The listing builds one solid part. Answer for the finished solid, in the listing's coordinates (mm). A direction names the side the tool comes from. Coordinates: 2 decimals unless noted, no trailing zeros. Order: outer loops, then holes, each group sorted by start corner. A loop starts at its lowest first (then second) coordinate and runs counter-clockwise, first axis right, second up. Notation, with made-up numbers: (-0.5, -6) -> (39.5, -6) arc R35 cw to (39.5, 31) -> close; hole circle Ø9 at (50.5, -33). An arc over 180 degrees is marked (long way). Write each question's results on one line, items separated by ' | '. Start each with the question number.
(1) The part is cut by section D-D, the plane x = -16. Give the vertices of the cut face in (y, z) (3 decimals).
(2) The part is cut by section C-C, the plane z = -17.5. Give the vertices of the cut face in (x, y).
(3) Given pin 1 (1.5 mm diameter, centred on x = 4, z = 4, fed in from +Y); pin 2 (7.5 mm diameter, centred on x = -5.5, y = -21, fed in from -Z) (3 decimals), each flat-ended and moving along its own axis, determine where each tip first touches the part or whether it passes through.
(4) The part is cut by section A-A, the plane z = 19.5. Give the vertices of the cut face in (x, y) (3 decimals).
(5) Determine the mould class of faces 1 (the face through (9.525, -32, 13)), 2 (the face through (-2, -31, 3.175)), 3 (the face through (0, -63.5, 0)) for opening direction Y: +Y half, -Y half, draft (parallel to the pull), parting line (faces both ways), or undercut.
(6) The part is cut by section B-B, the plane y = -51. Give the vertices of the cut face in (x, z) (3 decimals).
(7) A tool of negligible diameter and unlimited length cuts with its end or side. For faces 4 (the face through (-9.525, -8, 13)), 5 (the face through (-14, -47.625, 13)), 6 (the face through (-12.7, -32, -16)), from which of +Z, -Z, +X, -X, +Y, -Y can it reach the whole face along a straight path? Write none if from no direction.
(8) Straight lines are drawn through the part: L1, parallel to X at y = -31, z = -20; L2, parallel to X at y = -12, z = 3.5 (3 decimals); L3, parallel to Z at x = 4.5, y = -33 (3 decimals). For each, find the intervals that lie inside material, in ascending order.
```python
from build123d import *

# Parameters (mm, degrees)
F0_W     = 38.1
F0_H     = 44.45
F1_DEPTH = 63.5
F2_W     = 19.05
F2_H     = 19.05
F3_DEPTH = 63.501
F4_W     = 25.4
F4_H     = 12.7
F5_DEPTH = 63.501
F6_W     = 31.75
F6_H     = 19.05
F7_DEPTH = 9.525


with BuildPart() as f1:
    # F0 (on Front) → F1 (new body)
    with BuildSketch(Plane.XZ):
        Rectangle(F0_W, F0_H)
    extrude(amount=F1_DEPTH)

    # F2 (on face) → F3 (cut, through all)
    with BuildSketch(Plane.XZ.offset(63.5)):
        with Locations((0, 12.7)):
            Rectangle(F2_W, F2_H)
    extrude(amount=-F3_DEPTH, mode=Mode.SUBTRACT)

    # F4 (on face) → F5 (cut, through all)
    with BuildSketch(Plane.XZ.offset(63.5)):
        with Locations((0, -15.875)):
            Rectangle(F4_W, F4_H)
    extrude(amount=-F5_DEPTH, mode=Mode.SUBTRACT)

    # F6 (on face) → F7 (cut, through all)
    with BuildSketch(Plane(origin=(-19.05, 0, 0), x_dir=(0, -1, 0), z_dir=(-1, 0, 0))):
        with Locations((31.75, 12.7)):
            Rectangle(F6_W, F6_H)
    extrude(amount=-F7_DEPTH, mode=Mode.SUBTRACT)


solid = f1.part
```
Established:
1) outline: (-63.5, -22.225) -> (0, -22.225) -> (0, 22.225) -> (-15.875, 22.225) -> (-15.875, 3.175) -> (-47.625, 3.175) -> (-47.625, 22.225) -> (-63.5, 22.225) -> close
2) outline: (-19.05, -63.5) -> (-12.7, -63.5) -> (-12.7, 0) -> (-19.05, 0) -> close; (12.7, -63.5) -> (19.05, -63.5) -> (19.05, 0) -> (12.7, 0) -> close
3) pin 1: passes through | pin 2: stops at z = -9.525
4) outline: (-19.05, -63.5) -> (-9.525, -63.5) -> (-9.525, -47.625) -> (-19.05, -47.625) -> close; (-19.05, -15.875) -> (-9.525, -15.875) -> (-9.525, 0) -> (-19.05, 0) -> close; (9.525, -63.5) -> (19.05, -63.5) -> (19.05, 0) -> (9.525, 0) -> close
5) face 1: draft | face 2: undercut | face 3: -Y half
6) outline: (-19.05, -22.225) -> (-12.7, -22.225) -> (-12.7, -9.525) -> (12.7, -9.525) -> (12.7, -22.225) -> (19.05, -22.225) -> (19.05, 22.225) -> (9.525, 22.225) -> (9.525, 3.175) -> (-9.525, 3.175) -> (-9.525, 22.225) -> (-19.05, 22.225) -> close
7) face 4: +Z, +Y, -Y | face 5: +Z, -X | face 6: -Z, +Y, -Y
8) L1: x = -19.05 to -12.7, 12.7 to 19.05 | L2: x = -19.05 to -9.525, 9.525 to 19.05 | L3: z = -9.525 to 3.175
